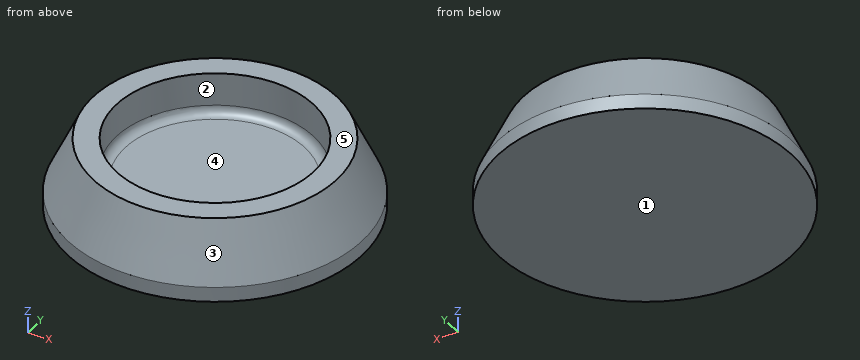
from build123d import *

# Parameters (mm, degrees)
F0_R     = 44.5
F1_DEPTH = 20
F1_TAPER = 25
F2_R     = 28.5
F3_DEPTH = 12
F4_R     = 44.5
F4_R_2   = 42.5
F5_DEPTH = 20.001
F6_R     = 2.5


with BuildPart() as f1:
    # F0 (on Top) → F1 (new body)
    with BuildSketch(Plane.XY):
        Circle(F0_R)
    extrude(amount=F1_DEPTH, taper=F1_TAPER)

    # F2 (on face) → F3 (cut)
    with BuildSketch(Plane.XY.offset(20)):
        Circle(F2_R)
    extrude(amount=-F3_DEPTH, mode=Mode.SUBTRACT)

    # F4 (on face) → F5 (cut, through all)
    with BuildSketch(Plane(origin=(0, 0, 0), x_dir=(1, 0, 0), z_dir=(0, 0, -1))):
        Circle(F4_R)
        Circle(F4_R_2, mode=Mode.SUBTRACT)
    extrude(amount=-F5_DEPTH, mode=Mode.SUBTRACT)

    # F6
    f6_edges = [f1.edges().sort_by_distance(p)[0] for p in [
        (-28.5, 0, 8),
    ]]
    fillet(f6_edges, radius=F6_R)


solid = f1.part
Here's how the part is built. I have some questions about the finished solid (model axes, mm). Face numbers are marked on the shaded views. A direction names the side the tool comes from. Give positions to 0.01 mm unless a question says otherwise; leave off trailing zeros. Loops run counter-clockwise (first coordinate to the right, second up) from the corner with the lowest first, then second, coordinate; pieces in that order, holes last. Notation, with made-up numbers: (47.5, 7.25) -> (81.5, 7.25) arc R34 cw to (81.5, 37.25) -> close; hole circle Ø3 at (25, -13.75). An arc over 180 degrees is marked (long way). One line per item, written item: value.
Q1. Suppose I cut it at C-C on z = 16.25. Please give me the cut outline in (x, y) (1 decimal).
Answers follow:
outline: circle Ø73.8 at (0, 0); hole circle Ø57 at (0, 0)
Q2. Suppose I cut it at D-D on z = 6. Please give me the cut outline in (x, y).
Answers follow:
outline: circle Ø83.4 at (0, 0)
Q3. Suppose I cut it at A-A on y = 0. Please give me the cut outline in (x, z), then the cut area to 3 significant figures.
Answers follow:
outline: (-42.5, 0) -> (42.5, 0) -> (42.5, 4.29) -> (35.17, 20) -> (28.5, 20) -> (28.5, 10.5) arc R2.5 cw to (26, 8) -> (-26, 8) arc R2.5 cw to (-28.5, 10.5) -> (-28.5, 20) -> (-35.17, 20) -> (-42.5, 4.29) -> close
area: 904 mm^2
Q4. I'm going to push flat-ended pins straight in: pin 1 Ø5 at (y, z) = (34, 12.5) entering from -X; pin 2 Ø6 at (y, z) = (21, 10.5) entering from -X; pin 3 Ø5 at (x, y) = (-20.5, -6) entering from +Z. Where does each tip first touch, or does it pass through?
Answers follow:
pin 1: x = -22.97
pin 2: x = -35.94
pin 3: z = 8
Q5. We'd pull the mould along Y, two halves only. Please class the marked faces 3, 4 and 5: pulls with the +Y half, pulls with the -Y half, needs draft (parallel to the pull), parting line crosses it, or undercut.
Answers follow:
face 3: parting line crosses it
face 4: undercut
face 5: needs draft
Q6. On a 3-axis mill with a long thin cutter (end or side, diameter ignored), from which of +Z, -Z, +X, -X, +Y, -Y can I reach the whole of each face in a straight line? I mean the marked faces 1 and 2. Say none if no direction works.
Answers follow:
face 1: -Z, +X, -X, +Y, -Y
face 2: +Z
Q7. If I drill on line 1 along Z through (x, y) = (-14, -14.5); line 2 along X through (y, z) = (-18, 15); line 3 along Z through (x, y) = (-8, -39), over which ranges is the centre line in solid material (lowest first)?
Answers follow:
line 1: 0 to 8
line 2: -32.9 to -22.1, 22.1 to 32.9
line 3: 0 to 10.05
